```python
from build123d import *

# Parameters (mm, degrees)
CROQUIS1_W                          = 30.988
CROQUIS1_H                          = 482.6
CROQUIS1_R                          = 3.9624
BRIDA_BASE1_DEPTH                   = 1.524
BRIDA_DE_ARISTA1_STRIP_W            = 9.144
BRIDA_DE_ARISTA1_STRIP_H            = 1.524
BRIDA_DE_ARISTA1_STRIP_CUT_DEPTH    = 438.15
BRIDA_DE_ARISTA1_RELIEF_W           = 9.2964
BRIDA_DE_ARISTA1_RELIEF_H           = 0.1524
BRIDA_DE_ARISTA1_RELIEF_CUT_DEPTH   = 1.524
BRIDA_DE_ARISTA1_STRIP_2_W          = 9.144
BRIDA_DE_ARISTA1_STRIP_2_H          = 1.524
BRIDA_DE_ARISTA1_STRIP_CUT_2_DEPTH  = 438.15
BRIDA_DE_ARISTA1_RELIEF_2_W         = 9.2964
BRIDA_DE_ARISTA1_RELIEF_2_H         = 0.1524
BRIDA_DE_ARISTA1_RELIEF_CUT_2_DEPTH = 1.524
BRIDA_DE_ARISTA1_DEPTH              = 438.15
BRIDA_DE_ARISTA1_BEND_DEPTH         = 438.15
CROQUIS15_R                         = 3.9624
CORTAR_EXTRUIR1_DEPTH               = 243.229986831


# Sheet-metal steps are written as plain solids
with BuildPart() as part:
    # Croquis1 → Brida base1 (new body)
    with BuildSketch(Plane.XY):
        Rectangle(CROQUIS1_W, CROQUIS1_H)
        with Locations((-0.508, 231.775)):
            Circle(CROQUIS1_R, mode=Mode.SUBTRACT)
        with Locations((0.508, -231.775)):
            Circle(CROQUIS1_R, mode=Mode.SUBTRACT)
    extrude(amount=-BRIDA_BASE1_DEPTH)

    # Brida de arista1 strip (across the edge) → Brida de arista1 strip cut (cut)
    with BuildSketch(Plane(origin=(15.494, -219.075, 0), x_dir=(-1, 0, 0), z_dir=(0, 1, 0))):
        with Locations((-1.524, -0.762)):
            Rectangle(BRIDA_DE_ARISTA1_STRIP_W, BRIDA_DE_ARISTA1_STRIP_H)
    extrude(amount=BRIDA_DE_ARISTA1_STRIP_CUT_DEPTH, mode=Mode.SUBTRACT)

    # Brida de arista1 relief (on the sheet) → Brida de arista1 relief cut (cut)
    with BuildSketch(Plane(origin=(12.446, -219.075, 0), x_dir=(-1, 0, 0), z_dir=(0, 0, 1))):
        with Locations((-4.4958, 0.0762)):
            Rectangle(BRIDA_DE_ARISTA1_RELIEF_W, BRIDA_DE_ARISTA1_RELIEF_H)
        with Locations((-4.4958, -438.2262)):
            Rectangle(BRIDA_DE_ARISTA1_RELIEF_W, BRIDA_DE_ARISTA1_RELIEF_H)
    extrude(amount=-BRIDA_DE_ARISTA1_RELIEF_CUT_DEPTH, mode=Mode.SUBTRACT)

    # Brida de arista1 strip 2 (across the edge) → Brida de arista1 strip cut 2 (cut)
    with BuildSketch(Plane(origin=(-15.494, 219.075, 0), x_dir=(1, 0, 0), z_dir=(0, -1, 0))):
        with Locations((-1.524, -0.762)):
            Rectangle(BRIDA_DE_ARISTA1_STRIP_2_W, BRIDA_DE_ARISTA1_STRIP_2_H)
    extrude(amount=BRIDA_DE_ARISTA1_STRIP_CUT_2_DEPTH, mode=Mode.SUBTRACT)

    # Brida de arista1 relief 2 (on the sheet) → Brida de arista1 relief cut 2 (cut)
    with BuildSketch(Plane(origin=(-12.446, 219.075, 0), x_dir=(1, 0, 0), z_dir=(0, 0, 1))):
        with Locations((-4.4958, 0.0762)):
            Rectangle(BRIDA_DE_ARISTA1_RELIEF_2_W, BRIDA_DE_ARISTA1_RELIEF_2_H)
        with Locations((-4.4958, -438.2262)):
            Rectangle(BRIDA_DE_ARISTA1_RELIEF_2_W, BRIDA_DE_ARISTA1_RELIEF_2_H)
    extrude(amount=-BRIDA_DE_ARISTA1_RELIEF_CUT_2_DEPTH, mode=Mode.SUBTRACT)

    # Brida de arista1 section (across the edge) → Brida de arista1 (add)
    with BuildSketch(Plane(origin=(15.494, -219.075, 0), x_dir=(-1, 0, 0), z_dir=(0, 1, 0))):
        with BuildLine():
            Line((0, 1.524), (0, 14.478))
            Line((0, 14.478), (1.524, 14.478))
            Line((1.524, 14.478), (1.524, 1.524))
            ThreePointArc((1.524, 1.524), (1.970369265, 0.446369265), (3.048, 0))
            Line((3.048, 0), (3.048, -1.524))
            ThreePointArc((3.048, -1.524), (0.892738531, -0.631261469), (0, 1.524))
        make_face()
    extrude(amount=BRIDA_DE_ARISTA1_DEPTH)

    # Brida de arista1 section 2 (across the edge) → Brida de arista1 bend (add)
    with BuildSketch(Plane(origin=(-15.494, 219.075, 0), x_dir=(1, 0, 0), z_dir=(0, -1, 0))):
        with BuildLine():
            Line((0, 1.524), (0, 14.478))
            Line((0, 14.478), (1.524, 14.478))
            Line((1.524, 14.478), (1.524, 1.524))
            ThreePointArc((1.524, 1.524), (1.970369265, 0.446369265), (3.048, 0))
            Line((3.048, 0), (3.048, -1.524))
            ThreePointArc((3.048, -1.524), (0.892738531, -0.631261469), (0, 1.524))
        make_face()
    extrude(amount=BRIDA_DE_ARISTA1_BEND_DEPTH)

    # Croquis15 → Cortar-Extruir1 (cut, through all)
    with BuildSketch(Plane.XY):
        with Locations((-15.9004, 231.775)):
            Circle(CROQUIS15_R)
        with Locations((-15.9004, -231.775)):
            Circle(CROQUIS15_R)
        with Locations((15.9004, -231.775)):
            Circle(CROQUIS15_R)
        with Locations((15.9004, 231.775)):
            Circle(CROQUIS15_R)
    extrude(amount=-CORTAR_EXTRUIR1_DEPTH, mode=Mode.SUBTRACT)


solid = part.part
```
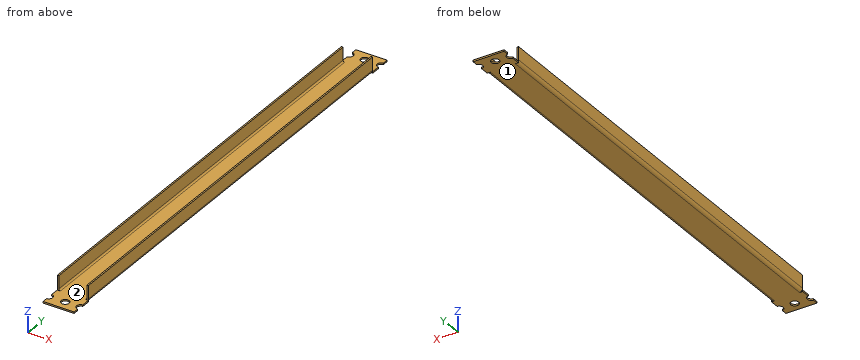
The model under review builds one solid part; all positions refer to its coordinate system, in mm. Face numbers are marked on the shaded views. Round coordinates to 2 decimals unless told otherwise and drop trailing zeros. Loops run counter-clockwise (first coordinate to the right, second up) from the corner with the lowest first, then second, coordinate; pieces in that order, holes last. Notation, with made-up numbers: M 71.5,36 L 87.5,36 A22 cw 87.5,68 Z; hole C -17.5,-26 d5. An arc over 180 degrees is marked long. Write item = value, one per line.
Item 1: Take a section at B-B on y = -190.5. Write out the cut boundary in (x, z).
Return value:
outline = M -15.49,1.52 A3.05 ccw -12.45,-1.52 L 12.45,-1.52 A3.05 ccw 15.49,1.52 L 15.49,14.48 L 13.97,14.48 L 13.97,1.52 A1.52 cw 12.45,0 L -12.45,0 A1.52 cw -13.97,1.52 L -13.97,14.48 L -15.49,14.48 Z
Item 2: The part is to be moulded in two halves that separate along X. For the marked faces 1 and 2, say which applies: released by +X, released by -X, zero draft, split by the parting line, or undercut.
Return value:
face_1 = zero draft
face_2 = undercut
Item 3: Insertion check: P1, Ø3, axis at x = 11, y = 108, coming from the +Z side; P2, Ø3.5, axis at x = 14.5, z = 10, coming from the +Y side (3 decimals); P3, Ø2.5, axis at x = 14, z = 8, coming from the -Y side (3 decimals). Each pin has a flat end and moves straight along its axis. Give the tip position at first contact, or say it passes through.
Return value:
P1 = 0
P2 = 219.075
P3 = -219.075
Item 4: Take a section at A-A on z = 8.75. Write out the cut boundary in (x, y) (3 decimals).
Return value:
outline = M -15.494,-219.075 L -13.97,-219.075 L -13.97,219.075 L -15.494,219.075 Z; M 13.97,-219.075 L 15.494,-219.075 L 15.494,219.075 L 13.97,219.075 Z
Item 5: For line 1 (X direction, y = -12, z = 3); line 2 (Z direction, x = -14, y = 221.5); line 3 (X direction, y = 158, z = 0.5), list the stretches that pass through material, from the lowest coordinate up. Write a range as [from, to].
Return value:
line_1 = [-15.49, -13.97], [13.97, 15.49]
line_2 = [-1.52, 0]
line_3 = [-15.32, -13.57], [13.57, 15.32]
